from build123d import *

# Parameters (mm, degrees)
SKETCH_1_W          = 64.5
SKETCH_1_H          = 45
EXTRUDE_1_DEPTH     = 3
HOLE_WIZARD_1_D     = 3.5
HOLE_WIZARD_2_D     = 15
SKETCH_7_W          = 64.5
SKETCH_7_H          = 5
EXTRUDE_2_DEPTH     = 37
HOLE_WIZARD_3_D     = 3.5
CUT_EXTRUDE_1_DEPTH = 3
EXTRUDE_3_DEPTH     = 3
SKETCH_15_W         = 65.5
SKETCH_15_H         = 37
CUT_EXTRUDE_2_DEPTH = 40


with BuildPart() as part:
    # 草图1 → 凸台-拉伸1 (new body)
    with BuildSketch(Plane.XY):
        with Locations((32.25, 22.5)):
            Rectangle(SKETCH_1_W, SKETCH_1_H)
    extrude(amount=EXTRUDE_1_DEPTH)

    # 孔1 (through all)
    with Locations(Plane.XY.offset(3)):
        with Locations((7.25, 39), (57.25, 39), (57.25, 12.5), (7.25, 12.5)):
            Hole(HOLE_WIZARD_1_D / 2)

    # 孔2 (through all)
    with Locations(Plane.XY.offset(3)):
        with Locations((12.9, 25.75), (51.6, 25.75)):
            Hole(HOLE_WIZARD_2_D / 2)

    # 草图7 → 凸台-拉伸2 (add)
    with BuildSketch(Plane.XY.offset(3)):
        with Locations((32.25, 2.5)):
            Rectangle(SKETCH_7_W, SKETCH_7_H)
    extrude(amount=EXTRUDE_2_DEPTH)

    # 孔3 (through all)
    with Locations(Plane(origin=(0, 0, 0), x_dir=(-1, 0, 0), z_dir=(0, -1, 0))):
        with Locations((-4.75, -34), (-4.75, -9), (-59.75, -9), (-59.75, -34)):
            Hole(HOLE_WIZARD_3_D / 2)

    # 草图11 → 切除-拉伸1 (cut)
    with BuildSketch(Plane(origin=(0, 5, 0), x_dir=(1, 0, 0), z_dir=(0, 1, 0))):
        Polygon((63.040896534, -9), (61.395448267, -6.15), (58.104551733, -6.15), (56.459103466, -9), (58.104551733, -11.85), (61.395448267, -11.85), align=None)
        Polygon((63.040896534, -34), (61.395448267, -31.15), (58.104551733, -31.15), (56.459103466, -34), (58.104551733, -36.85), (61.395448267, -36.85), align=None)
        Polygon((8.040896534, -34), (6.395448267, -31.15), (3.104551733, -31.15), (1.459103466, -34), (3.104551733, -36.85), (6.395448267, -36.85), align=None)
        Polygon((8.040896534, -9), (6.395448267, -6.15), (3.104551733, -6.15), (1.459103466, -9), (3.104551733, -11.85), (6.395448267, -11.85), align=None)
    extrude(amount=-CUT_EXTRUDE_1_DEPTH, mode=Mode.SUBTRACT)

    # 草图14 → 凸台-拉伸3 (add)
    with BuildSketch(Plane.ZY):
        Polygon((3, 45), (0, 45), (0, 0), (40, 0), (40, 5), (33.188933637, 5), (3, 5), (3, 37.636685013), align=None)
        Polygon((40, 5), (3, 45), (3, 37.636685013), (33.188933637, 5), align=None)
    extrude_3 = extrude(amount=EXTRUDE_3_DEPTH)

    # 镜向1: 凸台-拉伸3 across plane
    add(extrude_3.mirror(Plane.ZY.offset(-32.25)))

    # 草图15 → 切除-拉伸2 (cut)
    with BuildSketch(Plane(origin=(0, 5, 0), x_dir=(1, 0, 0), z_dir=(0, 1, 0))):
        with Locations((32.25, -21.5)):
            Rectangle(SKETCH_15_W, SKETCH_15_H)
    extrude(amount=CUT_EXTRUDE_2_DEPTH, mode=Mode.SUBTRACT)


solid = part.part
Verification items for the finished model (mm, model axes). A direction names the side the tool comes from. Give positions to 0.01 mm unless a question says otherwise; leave off trailing zeros. Loops run counter-clockwise (first coordinate to the right, second up) from the corner with the lowest first, then second, coordinate; pieces in that order, holes last.
1) Draft check along X on faces 1 (the cylindrical face through (61.419, 1.014, 8.474)), 2 (the flat face through (66.23, 24.72, 21.76)). Enter one of: pulls with the +X half, pulls with the -X half, needs draft (parallel to the pull), parting line crosses it, or undercut.
2) Set-up check for faces 3 (the flat face through (-1.73, 21.55, 17.88)), 4 (the cylindrical face through (3, 1, 34)), 5 (the flat face through (5, 4, 31.15)): record each of +Z, -Z, +X, -X, +Y, -Y from which the full face is reachable in a straight line by a thin tool's end or side.
3) Sectioned sample at C-C, the plane y = 4. Enter the section's corners in (x, z).
4) Sectioned sample at B-B, the plane x = 51.6. Enter the section's corners in (y, z), then the cut area to 3 significant figures.
5) Sectioned sample at A-A, the plane y = 39. Enter the section's corners in (x, z).
6) Depth check by flat-ended pin: pin 1 Ø12 at (x, y) = (33.5, 12.5) entering from +Z; pin 2 Ø6.5 at (x, z) = (61, 33.5) entering from +Y; pin 3 Ø1.7 at (x, z) = (3, 8.5) entering from +Y. Enter the tip coordinate at first touch or a pass-through.
7) Thickness scan on line 1 along X through (y, z) = (0.5, 34); line 2 along Y through (x, z) = (7, 1); line 3 along Z through (x, y) = (4.75, 0.8). Record the ranges inside material, lowest first.
8) Sectioned sample at D-D, the plane y = 12.5. Enter the section's corners in (x, z), then the cut area to 3 significant figures.
Answers:
1. face 1: undercut
1. face 2: needs draft
2. face 3: +X, -X
2. face 4: +Y, -Y
2. face 5: +Y
3. outline: (-3, 0) - (67.5, 0) - (67.5, 40) - (-3, 40) - close; hole (1.46, 9) - (3.1, 6.15) - (6.4, 6.15) - (8.04, 9) - (6.4, 11.85) - (3.1, 11.85) - close; hole (1.46, 34) - (3.1, 31.15) - (6.4, 31.15) - (8.04, 34) - (6.4, 36.85) - (3.1, 36.85) - close; hole (56.46, 9) - (58.1, 6.15) - (61.4, 6.15) - (63.04, 9) - (61.4, 11.85) - (58.1, 11.85) - close; hole (56.46, 34) - (58.1, 31.15) - (61.4, 31.15) - (63.04, 34) - (61.4, 36.85) - (58.1, 36.85) - close
4. outline: (0, 0) - (18.25, 0) - (18.25, 3) - (5, 3) - (5, 40) - (0, 40) - close; (33.25, 0) - (45, 0) - (45, 3) - (33.25, 3) - close
4. area: 275 mm2
5. outline: (-3, 0) - (5.5, 0) - (5.5, 3) - (-0.5, 3) - (-0.5, 8.55) - (-3, 8.55) - close; (9, 0) - (55.5, 0) - (55.5, 3) - (9, 3) - close; (59, 0) - (67.5, 0) - (67.5, 8.55) - (65, 8.55) - (65, 3) - (59, 3) - close
6. pin 1: stops at z = 3
6. pin 2: stops at y = 5
6. pin 3: stops at y = 2
7. line 1: x = -3 to 3, 6.5 to 58, 61.5 to 67.5
7. line 2: y = 0 to 10.77, 14.23 to 21.12, 30.38 to 37.27, 40.73 to 45
7. line 3: z = 0 to 7.25, 10.75 to 32.25, 35.75 to 40
8. outline: (-3, 0) - (5.5, 0) - (5.5, 3) - (-3, 3) - close; (-3, 26.25) - (-0.5, 26.25) - (-0.5, 33.06) - (-3, 33.06) - close; (9, 0) - (55.5, 0) - (55.5, 3) - (9, 3) - close; (59, 0) - (67.5, 0) - (67.5, 3) - (59, 3) - close; (65, 26.25) - (67.5, 26.25) - (67.5, 33.06) - (65, 33.06) - close
8. area: 225 mm2
